from build123d import *

# Parameters (mm, degrees)
CHAMFER1_SIZE = 0.5
FILLET1_R     = 0.5


with BuildPart() as part:
    # Sketch1 → Revolve1 (revolve)
    with BuildSketch(Plane.XY, mode=Mode.PRIVATE) as revolve1_sk:
        Polygon((0, 2.25), (0, 6), (2.540716612, 6), (2.540716612, 4.5), (10, 4.5), (10, 2.25), align=None)
    revolve(revolve1_sk.sketch.rotate(Axis((-1.743486548, 0, 0), (1, 0, 0)), 90), axis=Axis((-1.743486548, 0, 0), (1, 0, 0)))

    # Chamfer1
    chamfer1_edges = [part.edges().sort_by_distance(p)[0] for p in [
        (10, 0, -4.5),
        (0, 0, -6),
    ]]
    chamfer(chamfer1_edges, length=CHAMFER1_SIZE)

    # Fillet1
    fillet1_edges = [part.edges().sort_by_distance(p)[0] for p in [
        (2.540716612, 0, -4.5),
    ]]
    fillet(fillet1_edges, radius=FILLET1_R)


solid = part.part
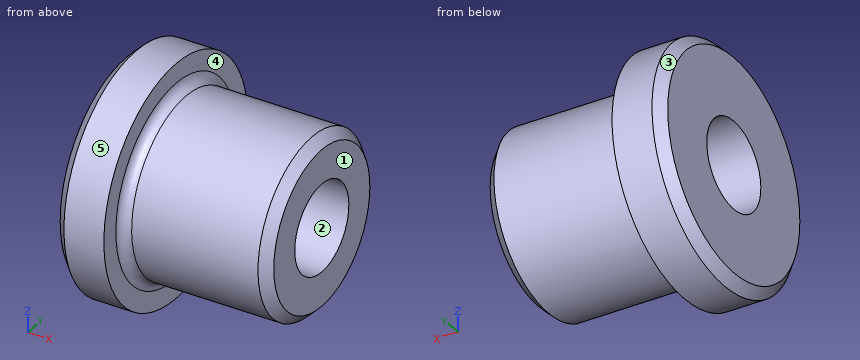
Input: part model. Units: mm. Frame: model coordinates. Face numbers are marked on the shaded views. A direction names the side the tool comes from. Coordinates: 2 decimals unless noted, no trailing zeros. Loops run counter-clockwise (first coordinate to the right, second up) from the corner with the lowest first, then second, coordinate; pieces in that order, holes last. Notation, with made-up numbers: (2.5, -38.75) -> (43.5, -38.75) arc R21 cw to (43.5, -3.75) -> close; hole circle Ø2 at (-3.75, 15). An arc over 180 degrees is marked (long way). One line per item, written item: value.
(1) Cut plane D-D (x = 2). Output: boundary loops of the cut face in (y, z), then the cut area to 3 significant figures.
Answer below:
outline: circle Ø12 at (0, 0); hole circle Ø4.5 at (0, 0)
area: 97.2 mm2
(2) Draft query along Z for the marked faces 1, 2 and 3. Return one class per face: pulls with the +Z half, pulls with the -Z half, needs draft (parallel to the pull), parting line crosses it, or undercut.
Answer below:
face 1: needs draft
face 2: undercut
face 3: parting line crosses it
(3) Ray query, line 1 along Y through (x, z) = (7.75, 0); line 2 along Y through (x, z) = (9.75, 1.5); line 3 along Z through (x, y) = (9, -1.5). Return the intervals inside material, ascending.
Answer below:
line 1: y = -4.5 to -2.25, 2.25 to 4.5
line 2: y = -3.98 to -1.68, 1.68 to 3.98
line 3: z = -4.24 to -1.68, 1.68 to 4.24
(4) Cut plane A-A (z = 0). Output: boundary loops of the cut face in (x, y), then the cut area to 3 significant figures.
Answer below:
outline: (0, -5.5) -> (0.5, -6) -> (2.54, -6) -> (2.54, -5) arc R0.5 cw to (3.04, -4.5) -> (9.5, -4.5) -> (10, -4) -> (10, -2.25) -> (0, -2.25) -> close; (0, 2.25) -> (10, 2.25) -> (10, 4) -> (9.5, 4.5) -> (3.04, 4.5) arc R0.5 cw to (2.54, 5) -> (2.54, 6) -> (0.5, 6) -> (0, 5.5) -> close
area: 52.2 mm2
(5) Pin query (flat end, axial travel): pin 1 Ø3.5 at (y, z) = (0, 0) entering from +X; pin 2 Ø4 at (x, z) = (4, -1.5) entering from +Y. Return the tip coordinate at first contact, or that it passes through.
Answer below:
pin 1: passes through
pin 2: stops at y = 6
(6) Cut plane C-C (x = 8.5). Output: boundary loops of the cut face in (y, z).
Answer below:
outline: circle Ø9 at (0, 0); hole circle Ø4.5 at (0, 0)
(7) Set-up query: the marked faces 4 and 5. Return all of +Z, -Z, +X, -X, +Y, -Y with unobstructed straight access to the full face (end or side cutting, diameter ignored); none if empty.
Answer below:
face 4: +X
face 5: +X, -X
